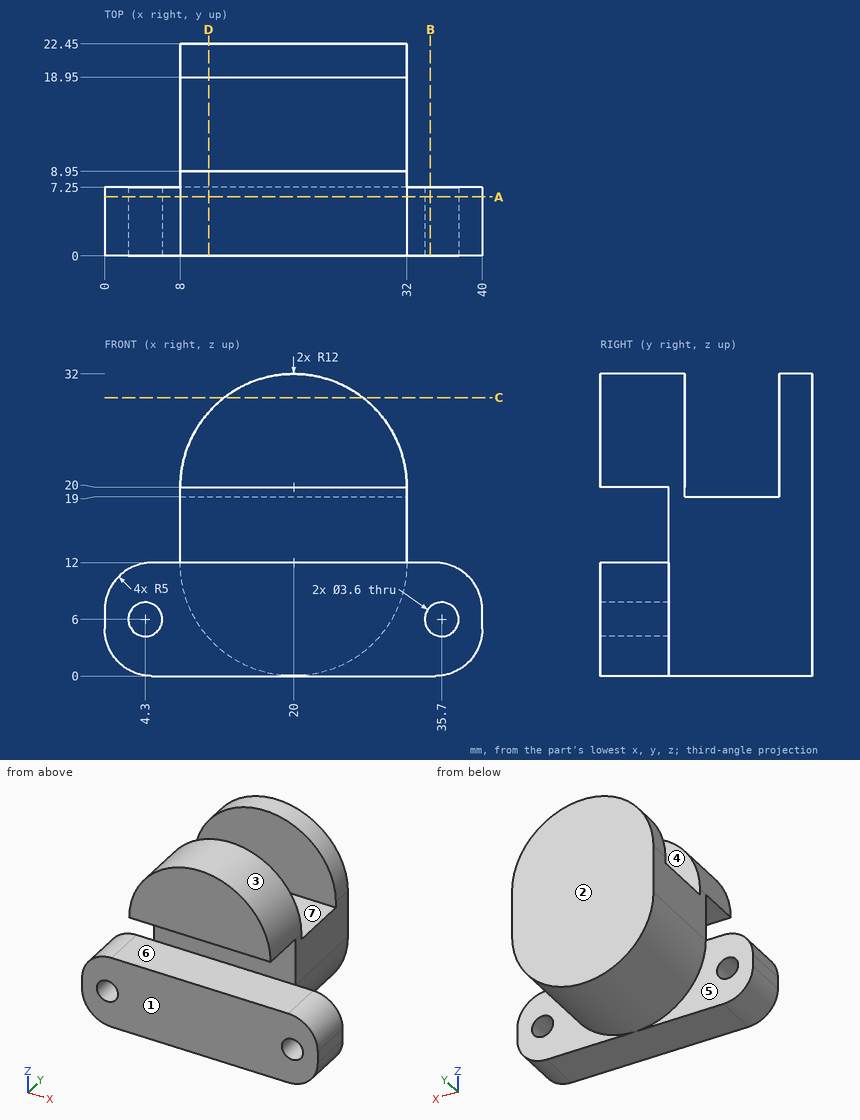
Answer from the drawing. Dimensions are ordinates in mm from the lowest x, y and z of the part. A direction names the side the tool comes from. Coordinates: 2 decimals unless noted, no trailing zeros. Loops run counter-clockwise (first coordinate to the right, second up) from the corner with the lowest first, then second, coordinate; pieces in that order, holes last. Notation, with made-up numbers: (-14, -16.75) - (28, -16.75) arc R9 ccw to (28, -0.75) - close; hole circle Ø5 at (2.25, -28). An arc over 180 degrees is marked (long way). Use a Markdown table: item, result.
Item 1: Given pin 1 Ø1.5 at (y, z) = (14, 13.5) entering from -X; pin 2 Ø5 at (x, z) = (30.5, 22) entering from -Y; pin 3 Ø4 at (x, y) = (9.5, 15.5) entering from +Z; pin 4 Ø4 at (y, z) = (17, 16.5) entering from +X, each flat-ended and moving along its own axis, determine where each tip first touches the part or whether it passes through.
Evaluation:
| item | result |
|---|---|
| pin 1 | stops at x = 8 |
| pin 2 | stops at y = 0 |
| pin 3 | stops at z = 19 |
| pin 4 | stops at x = 32 |
Item 2: Find section A-A, the plane y = 6.25. Determine the outline of the cut face in (x, z), and give its area (3 significant figures).
Evaluation:
| item | result |
|---|---|
| outline | (0, 5) arc R5 ccw to (5, 0) - (35, 0) arc R5 ccw to (40, 5) - (40, 7) arc R5 ccw to (35, 12) - (5, 12) arc R5 ccw to (0, 7) - close; (8, 20) - (32, 20) arc R12 ccw to start; hole circle Ø3.6 at (4.3, 6); hole circle Ø3.6 at (35.7, 6) |
| area | 664 mm2 |
Item 3: The mould has two halves that part along Y. Classify the marked faces 1, 2, 3 and 4: +Y half, -Y half, draft (parallel to the pull), parting line (faces both ways), or undercut.
Evaluation:
| item | result |
|---|---|
| face 1 | -Y half |
| face 2 | +Y half |
| face 3 | draft |
| face 4 | undercut |
Item 4: Find section D-D, the plane x = 11. Determine the outline of the cut face in (y, z).
Evaluation:
| item | result |
|---|---|
| outline | (0, 0) - (7.25, 0) - (7.25, 4.06) - (22.45, 4.06) - (22.45, 27.94) - (18.95, 27.94) - (18.95, 19) - (8.95, 19) - (8.95, 27.94) - (0, 27.94) - (0, 20) - (7.25, 20) - (7.25, 12) - (0, 12) - close |
Item 5: For the marked faces 5, 6 and 7, determine the directions among +Z, -Z, +X, -X, +Y, -Y from which every point of the face is accessible in a straight line to the end or side of a thin tool.
Evaluation:
| item | result |
|---|---|
| face 5 | -Z, -X, +Y |
| face 6 | +X, -X, -Y |
| face 7 | +Z, +X, -X |
Item 6: Find section B-B, the plane x = 34.5. Determine the outline of the cut face in (y, z), and give its area (3 significant figures).
Evaluation:
| item | result |
|---|---|
| outline | (0, 0) - (7.25, 0) - (7.25, 4.66) - (0, 4.66) - close; (0, 7.34) - (7.25, 7.34) - (7.25, 12) - (0, 12) - close |
| area | 67.5 mm2 |
Item 7: Find section C-C, the plane z = 29.5. Determine the outline of the cut face in (x, y), and give its area (3 significant figures).
Evaluation:
| item | result |
|---|---|
| outline | (12.67, 0) - (27.33, 0) - (27.33, 8.95) - (12.67, 8.95) - close; (12.67, 18.95) - (27.33, 18.95) - (27.33, 22.45) - (12.67, 22.45) - close |
| area | 183 mm2 |
Item 8: Consider probe 1 along Y at (x, z) = (10, 22); probe 2 along X at (y, z) = (2.5, 5.5); probe 3 along Z at (x, y) = (15.5, 2.25). Determine where each line is inside the solid, lowest interval first. Write a range as from..to.
Evaluation:
| item | result |
|---|---|
| probe 1 | y = 0..8.95, 18.95..22.45 |
| probe 2 | x = 0..2.57, 6.03..33.97, 37.43..40 |
| probe 3 | z = 0..12, 20..31.12 |
